from build123d import *

# Parameters (mm, degrees)
F0_W      = 59
F0_H      = 51.5
F1_DEPTH  = 26.8
F2_W      = 10
F2_H      = 8.65
F3_DEPTH  = 26.8
F4_W      = 1.5
F4_H      = 8.65
F5_DEPTH  = 22.75
F7_DEPTH  = 51.5
F9_DEPTH  = 51.5
F11_DEPTH = 51.5
F12_W     = 13
F12_H     = 3
F13_DEPTH = 5


with BuildPart() as f1:
    # F0 (on Top) → F1 (new body)
    with BuildSketch(Plane.XY):
        Rectangle(F0_W, F0_H)
    extrude(amount=F1_DEPTH)

    # F2 (on face) → F3 (cut)
    with BuildSketch(Plane.XY.offset(26.8)):
        with Locations((0, -21.425)):
            Rectangle(F2_W, F2_H)
    extrude(amount=-F3_DEPTH, mode=Mode.SUBTRACT)

    # F4 (on face) → F5 (cut)
    with BuildSketch(Plane.XY.offset(26.8)):
        with Locations((-5.75, -21.425)):
            Rectangle(F4_W, F4_H)
        with Locations((5.75, -21.425)):
            Rectangle(F4_W, F4_H)
    extrude(amount=-F5_DEPTH, mode=Mode.SUBTRACT)

    # F6 (on face) → F7 (cut)
    with BuildSketch(Plane.XZ.offset(25.75)):
        Polygon((-29.5, 26.8), (-29.5, 0), (-10.242246399, 26.8), align=None)
    extrude(amount=-F7_DEPTH, mode=Mode.SUBTRACT)

    # F8 (on face) → F9 (cut)
    with BuildSketch(Plane.XZ.offset(25.75)):
        Polygon((10.242246399, 26.8), (29.5, 0), (29.5, 26.8), align=None)
    extrude(amount=-F9_DEPTH, mode=Mode.SUBTRACT)

    # F10 (on face) → F11 (cut)
    with BuildSketch(Plane.XZ.offset(17.1)):
        Polygon((5, 8.67), (-5, 8.67), (-5, 4.05), (-5, 0), (5, 0), (5, 4.05), align=None)
    extrude(amount=-F11_DEPTH, mode=Mode.SUBTRACT)

    # F12 (on face) → F13 (cut)
    with BuildSketch(Plane.XZ.offset(17.1)):
        with Locations((0, 23.3)):
            Rectangle(F12_W, F12_H)
    extrude(amount=-F13_DEPTH, mode=Mode.SUBTRACT)


solid = f1.part
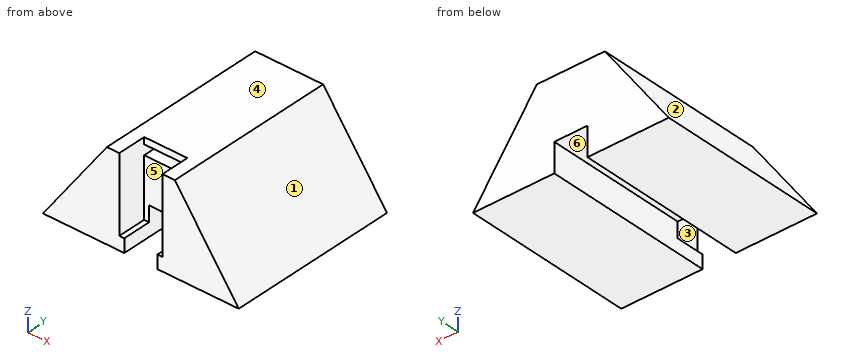
Read the model definition and answer for the solid it produces. Units are mm, in the model's axes. Face numbers are marked on the shaded views. A direction names the side the tool comes from. Round coordinates to 2 decimals unless told otherwise and drop trailing zeros. Order: outer loops, then holes, each group sorted by start corner. A loop starts at its lowest first (then second) coordinate and runs counter-clockwise, first axis right, second up.
1) The mould has two halves that part along X. Classify the marked faces 1, 2 and 3: released by +X, released by -X, zero draft, split by the parting line, or undercut.
2) The part is cut by section D-D on z = 18. Write down the section's boundary in (x, y), plus the area to 3 significant figures.
3) The part is cut by section A-A on z = 6.5. Write down the section's boundary in (x, y).
4) Flat-ended cylindrical pins translate along their axes: pin 1 (4.5 mm diameter, centred on y = -7, z = 4, fed in from -X); pin 2 (1.6 mm diameter, centred on x = 1.5, z = 26, fed in from -Y); pin 3 (3 mm diameter, centred on x = -1, y = 5, fed in from -Z). Find the tip coordinate at first contact, or state that the pin passes through.
5) For the marked faces 4, 5 and 6, determine the directions among +Z, -Z, +X, -X, +Y, -Y from which every point of the face is accessible in a straight line to the end or side of a thin tool.
6) The part is cut by section C-C on y = 2. Write down the section's boundary in (x, z), plus the area to 3 significant figures.
7) The part is cut by section B-B on y = -20.5. Write down the section's boundary in (x, z), plus the area to 3 significant figures.
8) Straight lines are drawn through the part: L1, parallel to Y at x = 6, z = 4.5; L2, parallel to Z at x = 2, y = 1; L3, parallel to X at y = -21, z = 22. For each, find the intervals that lie inside material, in ascending order.
Resolved:
1. face 1: released by +X
1. face 2: released by -X
1. face 3: undercut
2. outline: (-16.57, -25.75) - (-6.5, -25.75) - (-6.5, -17.1) - (6.5, -17.1) - (6.5, -25.75) - (16.57, -25.75) - (16.57, 25.75) - (-16.57, 25.75) - close
2. area: 1,590 mm2
3. outline: (-24.83, -25.75) - (-6.5, -25.75) - (-6.5, -17.1) - (-5, -17.1) - (-5, 25.75) - (-24.83, 25.75) - close; (5, -17.1) - (6.5, -17.1) - (6.5, -25.75) - (24.83, -25.75) - (24.83, 25.75) - (5, 25.75) - close
4. pin 1: stops at x = -28.24
4. pin 2: stops at y = -17.1
4. pin 3: stops at z = 8.67
5. face 4: +Z, +X, -X, +Y, -Y
5. face 5: +Z, -Y
5. face 6: -Z, +Y, -Y
6. outline: (-29.5, 0) - (-5, 0) - (-5, 8.67) - (5, 8.67) - (5, 0) - (29.5, 0) - (10.24, 26.8) - (-10.24, 26.8) - close
6. area: 978 mm2
7. outline: (-29.5, 0) - (-5, 0) - (-5, 4.05) - (-6.5, 4.05) - (-6.5, 26.8) - (-10.24, 26.8) - close; (5, 0) - (29.5, 0) - (10.24, 26.8) - (6.5, 26.8) - (6.5, 4.05) - (5, 4.05) - close
7. area: 729 mm2
8. L1: y = -17.1 to 25.75
8. L2: z = 8.67 to 26.8
8. L3: x = -13.69 to -6.5, 6.5 to 13.69
